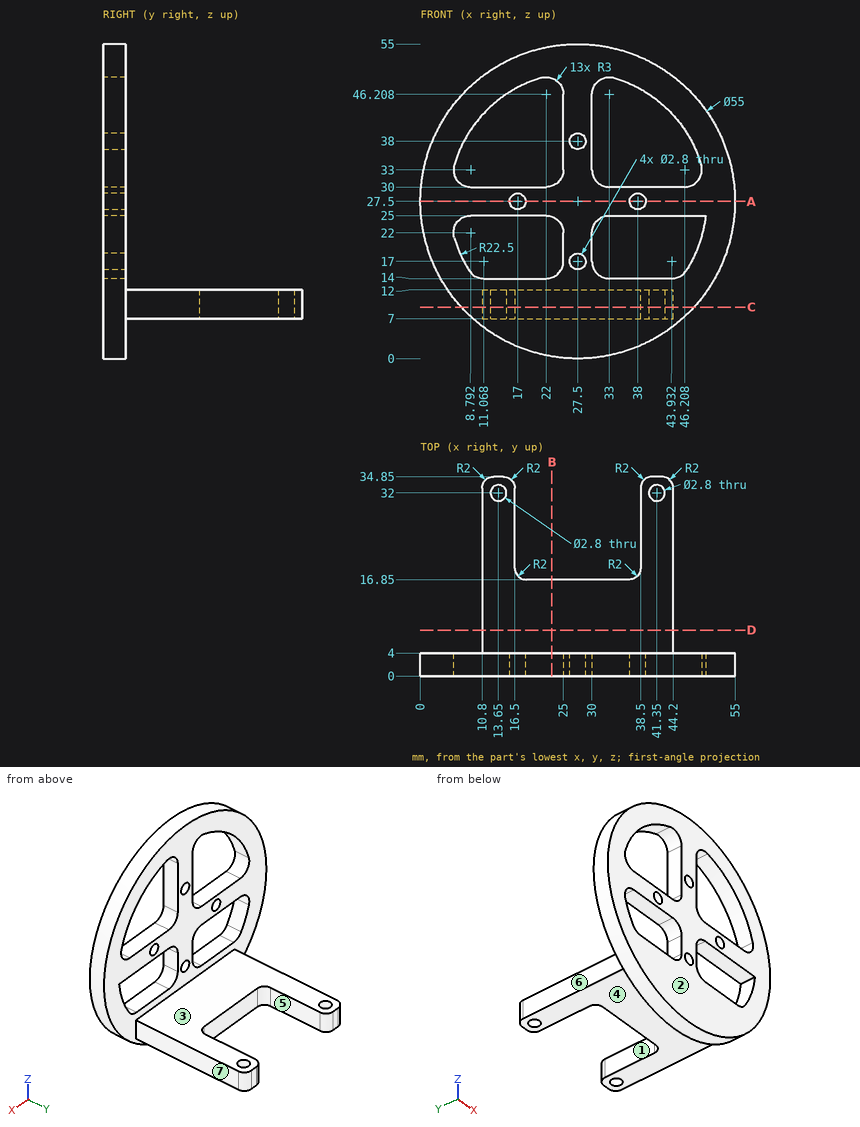
Input: dimensioned drawing with shaded views. Units: mm. Origin: part minimum x, y, z. A direction names the side the tool comes from. Give positions to 0.01 mm unless a question says otherwise; leave off trailing zeros. Write each loop counter-clockwise with the first axis right and the second up, starting at its lowest first coordinate (ties: lowest second). Pieces come first, ordered by that corner, then holes.
1. Draft query along X for the marked faces 5, 6 and 7. Return one class per face: released by +X, released by -X, zero draft, split by the parting line, or undercut.
2. Pin query (flat end, axial travel): P1, Ø3, axis at x = 38.5, y = 2, coming from the +Z side; P2, Ø3, axis at x = 39, y = 1.5, coming from the +Z side; P3, Ø4.5, axis at x = 18.5, y = 2.5, coming from the -Z side; P4, Ø1.7, axis at x = 17, z = 27.5, coming from the -Y side. Return the tip coordinate at first contact, or that it passes through.
3. Section query D-D, the plane y = 8. Return loops of the section in (x, z), then the cut area to 3 significant figures.
4. Line query: probe 1 along X at (y, z) = (2.9, 27.5); probe 2 along Z at (x, y) = (27, 3) (1 decimal); probe 3 along Z at (x, y) = (12.5, 2). Output: solid intervals per line, ascending.
5. Section query C-C, the plane z = 9. Return loops of the section in (x, y), then the cut area to 3 significant figures.
6. Section query A-A, the plane z = 27.5. Return loops of the section in (x, y).
7. Section query B-B, the plane x = 23. Return loops of the section in (y, z).
8. Reachability of the marked faces 1, 2, 3 and 4 from +Z, -Z, +X, -X, +Y, -Y: full face, straight path, thin tool, end or side. Return the list, or none.
Computed:
1. face 5: undercut
1. face 6: released by -X
1. face 7: released by +X
2. P1: stops at z = 53.31
2. P2: stops at z = 53.12
2. P3: stops at z = 0.84
2. P4: passes through
3. outline: (10.8, 7) - (44.2, 7) - (44.2, 12) - (10.8, 12) - close
3. area: 167 mm2
4. probe 1: x = 0 to 15.6, 18.4 to 36.6, 39.4 to 55
4. probe 2: z = 0 to 15.7, 18.3 to 36.7, 39.3 to 55
4. probe 3: z = 4.45 to 14, 25 to 30, 44.27 to 50.55
5. outline: (7.15, 0) - (47.85, 0) - (47.85, 4) - (44.2, 4) - (44.2, 32.85) arc R2 ccw to (42.2, 34.85) - (40.5, 34.85) arc R2 ccw to (38.5, 32.85) - (38.5, 18.85) arc R2 cw to (36.5, 16.85) - (18.5, 16.85) arc R2 cw to (16.5, 18.85) - (16.5, 32.85) arc R2 ccw to (14.5, 34.85) - (12.8, 34.85) arc R2 ccw to (10.8, 32.85) - (10.8, 4) - (7.15, 4) - close; hole circle Ø2.8 at (13.65, 32); hole circle Ø2.8 at (41.35, 32)
5. area: 783 mm2
6. outline: (0, 0) - (15.6, 0) - (15.6, 4) - (0, 4) - close; (18.4, 0) - (36.6, 0) - (36.6, 4) - (18.4, 4) - close; (39.4, 0) - (55, 0) - (55, 4) - (39.4, 4) - close
7. outline: (0, 0.37) - (4, 0.37) - (4, 7) - (16.85, 7) - (16.85, 12) - (4, 12) - (4, 14.17) - (0, 14.17) - close; (0, 24.83) - (4, 24.83) - (4, 30.17) - (0, 30.17) - close; (0, 49.04) - (4, 49.04) - (4, 54.63) - (0, 54.63) - close
8. face 1: +Z, -Z, +Y
8. face 2: +Z, -Z, +X, -X, -Y
8. face 3: +Z, +X, -X, +Y
8. face 4: -Z, +X, -X, +Y
